Can you work these out from the model? Positions are in its coordinate system, mm. Face numbers are marked on the shaded views. A direction names the side the tool comes from. Round coordinates to 2 decimals unless told otherwise and drop trailing zeros. Write each loop counter-clockwise with the first axis right and the second up, starting at its lowest first coordinate (ties: lowest second). Pieces come first, ordered by that corner, then holes. Notation, with made-up numbers: (-24, 88) -> (-1, 88) arc R15 ccw to (-1, 109) -> close; hole circle Ø9 at (-28.5, 28). An arc over 180 degrees is marked (long way). Write item = value, one per line. Start each with the question number.
1) Thinking about a two-plate mould opening in X: for the marked faces 3, 4 and 5, which applies, +X half, -X half, draft (parallel to the pull), parting line (faces both ways), or undercut?
2) For the marked faces 1 and 2, which set-ups out of +Z, -Z, +X, -X, +Y, -Y let a thin tool reach every point of the face, with its end or its side?
3) I'm going to push flat-ended pins straight in: pin 1 (2.5 mm diameter, centred on x = -23, z = 0, fed in from -Y); pin 2 (2 mm diameter, centred on x = -12, z = -20, fed in from -Y); pin 3 (1.5 mm diameter, centred on x = -2.5, y = -53.5, fed in from +Z). Where does each tip first touch, or does it pass through?
4) Imagine slicing it at B-B, the plane y = -23.5. Please give me the cut outline in (x, z).
5) If I drill on line 1 (Z direction, x = 16.5, y = -8.5); line 2 (Z direction, x = -23, y = -19); line 3 (X direction, y = -50.5, z = 1.5), over which ranges is the centre line in solid material (lowest first)?
6) Imagine slicing it at A-A, the plane z = 0. State how many separate pieces and enclosed holes the cut face has, then the cut area to 3 significant figures.
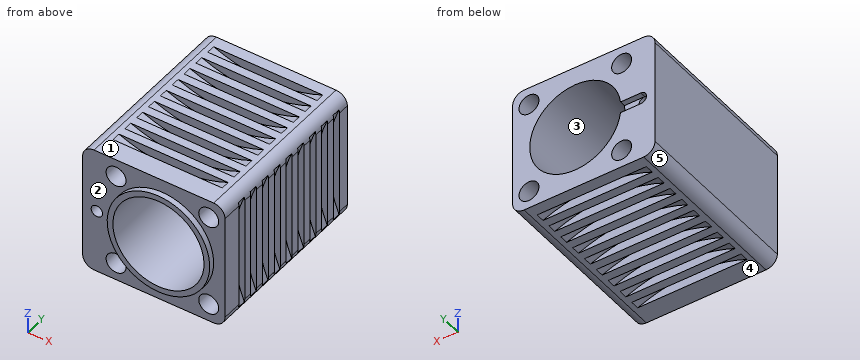
from build123d import *

# Parameters (mm, degrees)
BOSS_EXTRUDE1_DEPTH     = 62
SKETCH3_R               = 18
BOSS_EXTRUDE2_DEPTH     = 2
SKETCH4_R               = 16
CUT_EXTRUDE1_DEPTH      = 74.391075752
CUT_EXTRUDE2_DEPTH      = 2
SKETCH6_R               = 2
CUT_EXTRUDE3_DEPTH      = 72.653680994
SKETCH7_R               = 3.5
CUT_EXTRUDE4_DEPTH      = 74.391075752
SKETCH8_W               = 48
SKETCH8_H               = 3
LPATTERN1_COUNT         = 9
LPATTERN1_PITCH         = 6
MIRROR1_COPY_1_SKETCH_W = 48
MIRROR1_COPY_1_SKETCH_H = 3
MIRROR1_COPY_2_SKETCH_W = 48
MIRROR1_COPY_2_SKETCH_H = 3
MIRROR1_COPY_3_SKETCH_W = 48
MIRROR1_COPY_3_SKETCH_H = 3
MIRROR1_COPY_4_SKETCH_W = 48
MIRROR1_COPY_4_SKETCH_H = 3
MIRROR1_COPY_5_SKETCH_W = 48
MIRROR1_COPY_5_SKETCH_H = 3
MIRROR1_COPY_6_SKETCH_W = 48
MIRROR1_COPY_6_SKETCH_H = 3
MIRROR1_COPY_7_SKETCH_W = 48
MIRROR1_COPY_7_SKETCH_H = 3
MIRROR1_COPY_8_SKETCH_W = 48
MIRROR1_COPY_8_SKETCH_H = 3
SKETCH11_W              = 52.265084003
SKETCH11_H              = 3
LPATTERN2_COUNT         = 9
LPATTERN2_PITCH         = 6


with BuildPart() as part:
    # Sketch1 → Boss-Extrude1 (new body)
    with BuildSketch(Plane(origin=(0, 0, 0), x_dir=(1, 0, 0), z_dir=(0, 1, 0))):
        with BuildLine():
            Line((18, 22.5), (-24, 22.5))
            ThreePointArc((-24, 22.5), (-26.828427125, 21.328427125), (-28, 18.5))
            Line((-28, 18.5), (-28, -18.5))
            ThreePointArc((-28, -18.5), (-26.828427125, -21.328427125), (-24, -22.5))
            Line((-24, -22.5), (18, -22.5))
            ThreePointArc((18, -22.5), (20.828427125, -21.328427125), (22, -18.5))
            Line((22, -18.5), (22, 18.5))
            ThreePointArc((22, 18.5), (20.828427125, 21.328427125), (18, 22.5))
        make_face()
    extrude(amount=-BOSS_EXTRUDE1_DEPTH)

    # Sketch3 → Boss-Extrude2 (add)
    with BuildSketch(Plane.XZ.offset(62)):
        with Locations(Location((0, 0, 0), (0, 0, 270))):
            Circle(SKETCH3_R)
    extrude(amount=BOSS_EXTRUDE2_DEPTH)

    # Sketch4 → Cut-Extrude1 (cut, through all)
    with BuildSketch(Plane(origin=(0, 0, 0), x_dir=(1, 0, 0), z_dir=(0, 1, 0))):
        with Locations(Location((0, 0, 0), (0, 0, 270))):
            Circle(SKETCH4_R)
    extrude(amount=-CUT_EXTRUDE1_DEPTH, mode=Mode.SUBTRACT)

    # Sketch5 → Cut-Extrude2 (cut)
    with BuildSketch(Plane(origin=(0, 0, 0), x_dir=(1, 0, 0), z_dir=(0, 1, 0))):
        with BuildLine():
            Line((-23, 2), (-11, 2))
            ThreePointArc((-11, 2), (-9, 0), (-11, -2))
            Line((-11, -2), (-23, -2))
            ThreePointArc((-23, -2), (-25, 0), (-23, 2))
        make_face()
    extrude(amount=-CUT_EXTRUDE2_DEPTH, mode=Mode.SUBTRACT)

    # Sketch6 → Cut-Extrude3 (cut, through all)
    with BuildSketch(Plane(origin=(0, -2, 0), x_dir=(1, 0, 0), z_dir=(0, 1, 0))):
        with Locations(Location((-23, 0, 0), (0, 0, 270))):
            Circle(SKETCH6_R)
    extrude(amount=-CUT_EXTRUDE3_DEPTH, mode=Mode.SUBTRACT)

    # Sketch7 → Cut-Extrude4 (cut, through all)
    with BuildSketch(Plane(origin=(0, 0, 0), x_dir=(1, 0, 0), z_dir=(0, 1, 0))):
        with Locations(Location((16.263455967, 16.263455967, 0), (0, 0, 270))):
            Circle(SKETCH7_R)
        with Locations(Location((16.263455967, -16.263455967, 0), (0, 0, 270))):
            Circle(SKETCH7_R)
        with Locations(Location((-16.263455967, -16.263455967, 0), (0, 0, 270))):
            Circle(SKETCH7_R)
        with Locations(Location((-16.263455967, 16.263455967, 0), (0, 0, 270))):
            Circle(SKETCH7_R)
    extrude(amount=-CUT_EXTRUDE4_DEPTH, mode=Mode.SUBTRACT)

    # Sketch8 → Cut-Revolve1 (revolve, cut)
    with BuildSketch(Plane(origin=(-3, 0, 0), x_dir=(0, 0, -1), z_dir=(1, 0, 0))):
        with Locations((-42.5, -5.5)):
            Rectangle(SKETCH8_W, SKETCH8_H)
    cut_revolve1 = revolve(axis=Axis((-3, -4, 66.5), (0, -1, 0)), mode=Mode.SUBTRACT)

    # LPattern1: Cut-Revolve1 ×9
    with Locations(*[(0, -i * LPATTERN1_PITCH, 0) for i in range(1, LPATTERN1_COUNT)]):
        add(cut_revolve1, mode=Mode.SUBTRACT)

    # Mirror1: Cut-Revolve1 across plane
    add(cut_revolve1.mirror(Plane.XY), mode=Mode.SUBTRACT)

    # Mirror1 copy 1 sketch → Mirror1 copy 1 (revolve, cut)
    with BuildSketch(Plane(origin=(-3, -6, 0), x_dir=(0, 0, 1), z_dir=(1, 0, 0))):
        with Locations((-42.5, 5.5)):
            Rectangle(MIRROR1_COPY_1_SKETCH_W, MIRROR1_COPY_1_SKETCH_H)
    revolve(axis=Axis((-3, -10, -66.5), (0, 1, 0)), mode=Mode.SUBTRACT)

    # Mirror1 copy 2 sketch → Mirror1 copy 2 (revolve, cut)
    with BuildSketch(Plane(origin=(-3, -12, 0), x_dir=(0, 0, 1), z_dir=(1, 0, 0))):
        with Locations((-42.5, 5.5)):
            Rectangle(MIRROR1_COPY_2_SKETCH_W, MIRROR1_COPY_2_SKETCH_H)
    revolve(axis=Axis((-3, -16, -66.5), (0, 1, 0)), mode=Mode.SUBTRACT)

    # Mirror1 copy 3 sketch → Mirror1 copy 3 (revolve, cut)
    with BuildSketch(Plane(origin=(-3, -18, 0), x_dir=(0, 0, 1), z_dir=(1, 0, 0))):
        with Locations((-42.5, 5.5)):
            Rectangle(MIRROR1_COPY_3_SKETCH_W, MIRROR1_COPY_3_SKETCH_H)
    revolve(axis=Axis((-3, -22, -66.5), (0, 1, 0)), mode=Mode.SUBTRACT)

    # Mirror1 copy 4 sketch → Mirror1 copy 4 (revolve, cut)
    with BuildSketch(Plane(origin=(-3, -24, 0), x_dir=(0, 0, 1), z_dir=(1, 0, 0))):
        with Locations((-42.5, 5.5)):
            Rectangle(MIRROR1_COPY_4_SKETCH_W, MIRROR1_COPY_4_SKETCH_H)
    revolve(axis=Axis((-3, -28, -66.5), (0, 1, 0)), mode=Mode.SUBTRACT)

    # Mirror1 copy 5 sketch → Mirror1 copy 5 (revolve, cut)
    with BuildSketch(Plane(origin=(-3, -30, 0), x_dir=(0, 0, 1), z_dir=(1, 0, 0))):
        with Locations((-42.5, 5.5)):
            Rectangle(MIRROR1_COPY_5_SKETCH_W, MIRROR1_COPY_5_SKETCH_H)
    revolve(axis=Axis((-3, -34, -66.5), (0, 1, 0)), mode=Mode.SUBTRACT)

    # Mirror1 copy 6 sketch → Mirror1 copy 6 (revolve, cut)
    with BuildSketch(Plane(origin=(-3, -36, 0), x_dir=(0, 0, 1), z_dir=(1, 0, 0))):
        with Locations((-42.5, 5.5)):
            Rectangle(MIRROR1_COPY_6_SKETCH_W, MIRROR1_COPY_6_SKETCH_H)
    revolve(axis=Axis((-3, -40, -66.5), (0, 1, 0)), mode=Mode.SUBTRACT)

    # Mirror1 copy 7 sketch → Mirror1 copy 7 (revolve, cut)
    with BuildSketch(Plane(origin=(-3, -42, 0), x_dir=(0, 0, 1), z_dir=(1, 0, 0))):
        with Locations((-42.5, 5.5)):
            Rectangle(MIRROR1_COPY_7_SKETCH_W, MIRROR1_COPY_7_SKETCH_H)
    revolve(axis=Axis((-3, -46, -66.5), (0, 1, 0)), mode=Mode.SUBTRACT)

    # Mirror1 copy 8 sketch → Mirror1 copy 8 (revolve, cut)
    with BuildSketch(Plane(origin=(-3, -48, 0), x_dir=(0, 0, 1), z_dir=(1, 0, 0))):
        with Locations((-42.5, 5.5)):
            Rectangle(MIRROR1_COPY_8_SKETCH_W, MIRROR1_COPY_8_SKETCH_H)
    revolve(axis=Axis((-3, -52, -66.5), (0, 1, 0)), mode=Mode.SUBTRACT)

    # Sketch11 → Cut-Revolve3 (revolve, cut)
    with BuildSketch(Plane.XY):
        with Locations((44.132542001, -5.5)):
            Rectangle(SKETCH11_W, SKETCH11_H)
    cut_revolve3 = revolve(axis=Axis((70.265084003, -4, 0), (0, -1, 0)), mode=Mode.SUBTRACT)

    # LPattern2: Cut-Revolve3 ×9
    with Locations(*[(0, -i * LPATTERN2_PITCH, 0) for i in range(1, LPATTERN2_COUNT)]):
        add(cut_revolve3, mode=Mode.SUBTRACT)


solid = part.part
Reported:
q1.face_3 = undercut
q1.face_4 = draft
q1.face_5 = -X half
q2.face_1 = +Z, +X, -X, +Y, -Y
q2.face_2 = -Y
q3.pin_1 = through
q3.pin_2 = -62
q3.pin_3 = 18.52
q4.outline = (-28, -18.5) arc R4 ccw to (-24, -22.5) -> (-22.18, -22.5) arc R48 cw to (16.18, -22.5) -> (18, -22.5) arc R4 ccw to (21.83, -19.65) arc R52.27 cw to (21.83, 19.65) arc R4 ccw to (18, 22.5) -> (16.18, 22.5) arc R48 cw to (-22.18, 22.5) -> (-24, 22.5) arc R4 ccw to (-28, 18.5) -> close; hole circle Ø4 at (-23, 0); hole circle Ø7 at (-16.26, -16.26); hole circle Ø7 at (-16.26, 16.26); hole circle Ø32 at (0, 0); hole circle Ø7 at (16.26, -16.26); hole circle Ø7 at (16.26, 16.26)
q5.line_1 = -22.5 to -19.76, -12.77 to 12.77, 19.76 to 22.5
q5.line_2 = -22.5 to -2, 2 to 22.5
q5.line_3 = -28 to -24.32, -21.68 to -15.93, 15.93 to 22
q6.separate_pieces = 3
q6.enclosed_holes = 0
q6.area = 758 mm²
